Geometry: see drawing. Coordinates: mm, zero at the bounding-box minimum. Coordinates: 2 decimals unless noted, no trailing zeros. Order: outer loops, then holes, each group sorted by start corner. A loop starts at its lowest first (then second) coordinate and runs counter-clockwise, first axis right, second up. Notation, with made-up numbers: (38.25, -24.5) - (72.25, -24.5) arc R23 cw to (72.25, 13.5) - close; hole circle Ø11 at (88.5, 80). An arc over 180 degrees is marked (long way). Use a Markdown table: item, result. Add a question column.
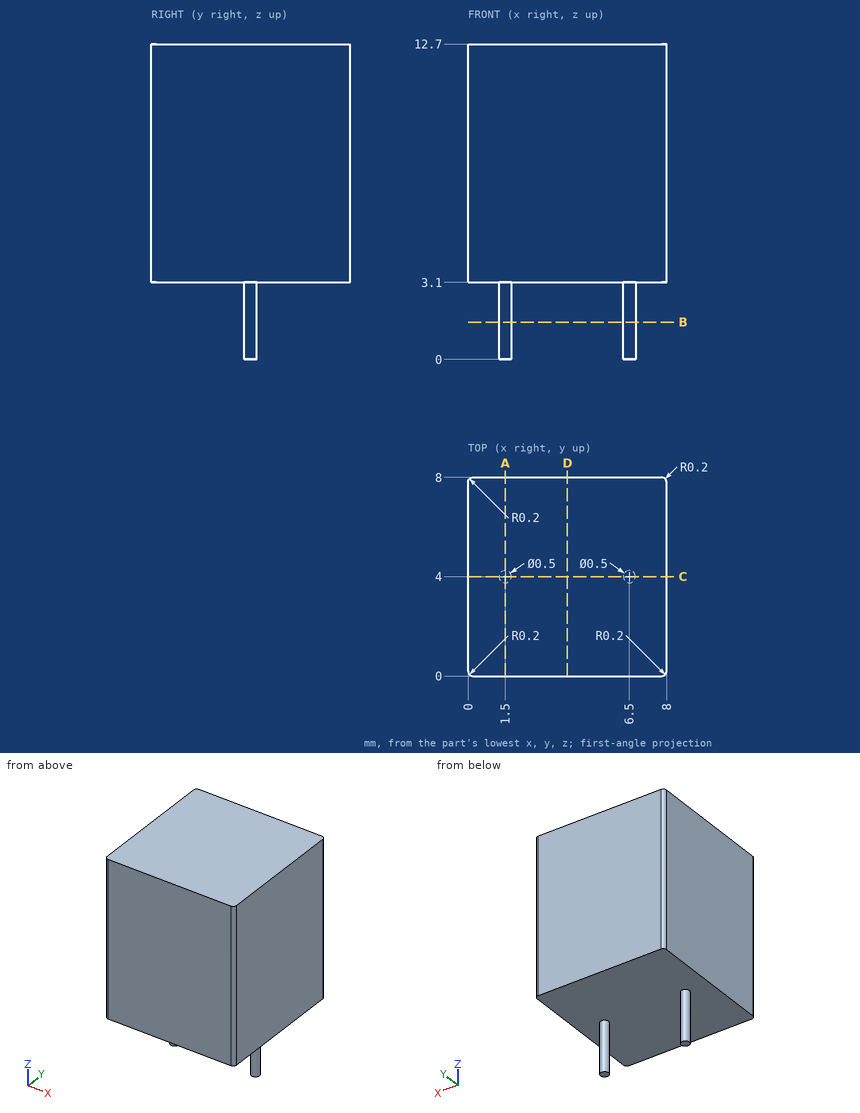
1) Section query B-B (z = 1.5). Return the cut outline in (x, y).
2) First-contact query: pin 1 (1.5 mm diameter, centred on x = 6.5, y = 6, fed in from -Z). Flat tip, straight axial feed; report the tip coordinate or a pass-through.
3) Section query A-A (x = 1.5). Return the cut outline in (y, z), and give its area (4 significant figures).
4) Line query: line 1 (Z direction, x = 0.5, y = 7). Output: solid intervals per line, ascending. Write a range as from..to.
5) Section query D-D (x = 4). Return the cut outline in (y, z), and give its area (3 significant figures).
6) Section query C-C (y = 4). Return the cut outline in (x, z), and give its area (3 significant figures).
From the geometry:
| question | item | result |
|---|---|---|
| 1 | outline | circle Ø0.5 at (1.5, 4); circle Ø0.5 at (6.5, 4) |
| 2 | pin 1 | stops at z = 3.1 |
| 3 | outline | (0, 3.1) - (3.75, 3.1) - (3.75, 0) - (4.25, 0) - (4.25, 3.1) - (8, 3.1) - (8, 12.7) - (0, 12.7) - close |
| 3 | area | 78.35 mm^2 |
| 4 | line 1 | z = 3.1..12.7 |
| 5 | outline | (0, 3.1) - (8, 3.1) - (8, 12.7) - (0, 12.7) - close |
| 5 | area | 76.8 mm^2 |
| 6 | outline | (0, 3.1) - (1.25, 3.1) - (1.25, 0) - (1.75, 0) - (1.75, 3.1) - (6.25, 3.1) - (6.25, 0) - (6.75, 0) - (6.75, 3.1) - (8, 3.1) - (8, 12.7) - (0, 12.7) - close |
| 6 | area | 79.9 mm^2 |
